Check sheet for the modelled part. Datum: model origin and axes. Units: mm. Coordinates: 2 decimals unless noted, no trailing zeros. Loops run counter-clockwise (first coordinate to the right, second up) from the corner with the lowest first, then second, coordinate; pieces in that order, holes last. Notation, with made-up numbers: (-10.75, 10) -> (19.25, 10) arc R6 cw to (19.25, 21) -> close; hole circle Ø5 at (11, 35). An arc over 180 degrees is marked (long way). Use one line per item in the form item = value.
from build123d import *

# Parameters (mm, degrees)
F4_R = 20


with BuildPart() as f1:
    # F0 (on Front) → F1 (revolve)
    with BuildSketch(Plane.XZ):
        with BuildLine():
            Line((0, -50), (0, 50))
            ThreePointArc((0, 50), (-50, 0), (0, -50))
        make_face()
    revolve(axis=Axis((0, 0, 0), (0, 0, -1)))

    # F3: F1 across plane


with BuildPart() as f1_1:
    add(f1.part)
    add(f1.part.mirror(Plane.XY.offset(40)))

    # F4
    f4_edges = [f1_1.edges().sort_by_distance(p)[0] for p in [
        (30, 0, 40),
        (-47.434165, 0, -15.811388),
    ]]
    fillet(f4_edges, radius=F4_R)


solid = f1_1.part
(1) Section check B-B, the plane z = 70. Record the boundary of the cut face in (x, y), plus the area to 3 significant figures.
Established:
outline = circle Ø97.98 at (0, 0)
area = 7,540 mm²
(2) Scan lines: line 1 along Z through (x, y) = (-35.5, 30); line 2 along Z through (x, y) = (-39, -18); line 3 along Z through (x, y) = (-6, 32). Record each from-to range of solid material in increasing order.
Established:
line_1 = -18.43 to 18.43, 61.57 to 98.43
line_2 = -25.59 to 25.59, 54.41 to 105.59
line_3 = -37.95 to 117.95
(3) Section check A-A, the plane z = 105. Record the boundary of the cut face in (x, y).
Established:
outline = circle Ø86.6 at (0, 0)
(4) Go/stop test with flat-tipped pins: P1, Ø8, axis at y = -9.5, z = 2, coming from the -X side; P2, Ø1.5, axis at x = 19.5, y = 20.5, coming from the -Z side; P3, Ø12, axis at x = 2.5, y = 0, coming from the -Z side; P4, Ø4, axis at x = 29.5, y = -11.5, coming from the -Z side. Record where each tip stops, or that it passes through.
Established:
P1 = -49.67
P2 = -41.73
P3 = -50
P4 = -40.25
